Input: part model. Units: mm. Frame: model coordinates. A direction names the side the tool comes from. Coordinates: 2 decimals unless noted, no trailing zeros. Order: outer loops, then holes, each group sorted by start corner. A loop starts at its lowest first (then second) coordinate and runs counter-clockwise, first axis right, second up. Notation, with made-up numbers: (16.25, -23.5) - (41.25, -23.5) arc R18 ccw to (41.25, -14.5) - close; hole circle Ø2 at (6, -6). An arc over 180 degrees is marked (long way). Answer as CSV lines item,"result". Start each with the question number.
Item 1: Material intervals for line 1 along X through (y, z) = (-8.5, 14); line 2 along Z through (x, y) = (16, -13) (3 decimals); line 3 along X through (y, z) = (-14.5, 21.5), sorted ascending.
Item 2: First-contact query: pin 1 (0.8 mm diameter, centred on x = 45, z = 11.5, fed in from -Y); pin 2 (1.9 mm diameter, centred on x = 46, y = -16, fed in from -Z); pin 3 (0.8 mm diameter, centred on x = 18.5, z = 23, fed in from -Y). Flat tips, straight axial feed; report the tip coordinate or a pass-through.
Item 3: Section D-D (y = -11). Output: boundary loops of the cut face in (x, z) (3 decimals), and give its area (3 significant figures).
Item 4: Section A-A (x = 17). Output: boundary loops of the cut face in (y, z) (3 decimals).
Item 5: Section C-C (y = 8.5). Output: boundary loops of the cut face in (x, z) (3 decimals).
Item 6: Draft query along Y for faces 6 (the flat face through (46, 15.13, 11)), 7 (the flat face through (46, 16.864, 11)), 8 (the flat face through (-1, -9.963, 23)). Return one class per face: +Y half, -Y half, draft (parallel to the pull), parting line (faces both ways), or undercut.
Item 7: Access query for faces 1 (the flat face through (-1, 9.747, 23)), 2 (the flat face through (46.99, 16, 11)), 3 (the flat face through (46, -16.864, 11)), 4 (the flat face through (46, -16, 6.35)), 5 (the flat face through (40.652, 0, 23)). Directions: +Z, -Z, +X, -X, +Y, -Y. A direction counts if a zero-diameter tool reaches every point of the face in a straight line with its end or side. Return the directions, or none.
Item 8: Section B-B (z = 10.75). Output: boundary loops of the cut face in (x, y) (3 decimals).
from build123d import *

# Parameters (mm, degrees)
SKETCH1_W           = 88.9
SKETCH1_H           = 34.29
BOSS_EXTRUDE1_DEPTH = 22.225
FILLET1_R           = 2.54
SKETCH2_W           = 9.52578488
SKETCH2_H           = 1.733476194
BOSS_EXTRUDE2_DEPTH = 2.54
SKETCH3_W           = 81.632090284
SKETCH3_H           = 19.709925483
BOSS_EXTRUDE3_DEPTH = 2.54


with BuildPart() as part:
    # Sketch1 → Boss-Extrude1 (new body)
    with BuildSketch(Plane.XY):
        Rectangle(SKETCH1_W, SKETCH1_H)
    extrude(amount=BOSS_EXTRUDE1_DEPTH)

    # Fillet1
    fillet1_edges = [part.edges().sort_by_distance(p)[0] for p in [
        (-44.45, 0, 22.225),
        (44.45, 0, 22.225),
        (-44.45, 0, 0),
        (44.45, 0, 0),
    ]]
    fillet(fillet1_edges, radius=FILLET1_R)

    # Sketch2 → Boss-Extrude2 (add)
    with BuildSketch(Plane(origin=(44.45, 0, 0), x_dir=(0, 0, -1), z_dir=(1, 0, 0))):
        with Locations((-11.1125, 15.996812485)):
            Rectangle(SKETCH2_W, SKETCH2_H)
    boss_extrude2 = extrude(amount=BOSS_EXTRUDE2_DEPTH)

    # Mirror1: Boss-Extrude2 across plane
    add(boss_extrude2.mirror(Plane.ZX))

    # Sketch3 → Boss-Extrude3 (add)
    with BuildSketch(Plane.XY.offset(22.225)):
        with Locations((-0.163591475, -0.108131836)):
            Rectangle(SKETCH3_W, SKETCH3_H)
    extrude(amount=BOSS_EXTRUDE3_DEPTH)


solid = part.part
Determined:
1,line 1,"x = -44.45 to 44.45"
1,line 2,"z = 0 to 22.225"
1,line 3,"x = -43.69 to 43.69"
2,pin 1,"stops at y = -16.86"
2,pin 2,"stops at z = 6.35"
2,pin 3,"stops at y = -9.96"
3,outline,"(-44.45, 2.54) arc R2.54 ccw to (-41.91, 0) - (41.91, 0) arc R2.54 ccw to (44.45, 2.54) - (44.45, 19.685) arc R2.54 ccw to (41.91, 22.225) - (-41.91, 22.225) arc R2.54 ccw to (-44.45, 19.685) - close"
3,area,"1,970 mm^2"
4,outline,"(-17.145, 0) - (17.145, 0) - (17.145, 22.225) - (9.747, 22.225) - (9.747, 24.765) - (-9.963, 24.765) - (-9.963, 22.225) - (-17.145, 22.225) - close"
5,outline,"(-44.45, 2.54) arc R2.54 ccw to (-41.91, 0) - (41.91, 0) arc R2.54 ccw to (44.45, 2.54) - (44.45, 19.685) arc R2.54 ccw to (41.91, 22.225) - (40.652, 22.225) - (40.652, 24.765) - (-40.98, 24.765) - (-40.98, 22.225) - (-41.91, 22.225) arc R2.54 ccw to (-44.45, 19.685) - close"
6,face 6,"undercut"
6,face 7,"+Y half"
6,face 8,"-Y half"
7,face 1,"+Z, +X, -X, +Y"
7,face 2,"+Z, -Z, +X, +Y, -Y"
7,face 3,"+Z, -Z, +X, -Y"
7,face 4,"-Z, +X, +Y, -Y"
7,face 5,"+Z, +X, +Y, -Y"
8,outline,"(-44.45, -17.145) - (44.45, -17.145) - (44.45, -16.864) - (46.99, -16.864) - (46.99, -15.13) - (44.45, -15.13) - (44.45, 15.13) - (46.99, 15.13) - (46.99, 16.864) - (44.45, 16.864) - (44.45, 17.145) - (-44.45, 17.145) - close"
